Verification items for the finished model (mm, model axes). Coordinates: 2 decimals unless noted, no trailing zeros. Order: outer loops, then holes, each group sorted by start corner. A loop starts at its lowest first (then second) coordinate and runs counter-clockwise, first axis right, second up.
Q1. Thickness scan on line 1 (X direction, y = -157.5, z = 1.6); line 2 (X direction, y = -42, z = 1.55). Record the ranges inside material, lowest first.
Q2. Cross-section at A-A, the plane y = -42.5. Record the boundary of the cut face in (x, z) (3 decimals).
Q3. Cross-section at B-B, the plane x = 138. Record the boundary of the cut face in (y, z) (3 decimals), and give its area (3 significant figures).
from build123d import *

# Parameters (mm, degrees)
SKETCH1_W           = 166.124
SKETCH1_H           = 207.09
SKETCH1_R           = 3.175
BOSS_EXTRUDE1_DEPTH = 3.175


with BuildPart() as part:
    # Sketch1 → Boss-Extrude1 (new body)
    with BuildSketch(Plane.XY):
        with Locations((83.062, -103.545)):
            Rectangle(SKETCH1_W, SKETCH1_H)
        with Locations((28.287, -42.5)):
            Circle(SKETCH1_R, mode=Mode.SUBTRACT)
        with Locations(Location((137.837, -42.5, 0), (0, 0, 180))):
            Circle(SKETCH1_R, mode=Mode.SUBTRACT)
        with Locations(Location((28.287, -157.5, 0), (0, 0, 180))):
            Circle(SKETCH1_R, mode=Mode.SUBTRACT)
        with Locations((137.837, -157.5)):
            Circle(SKETCH1_R, mode=Mode.SUBTRACT)
    extrude(amount=BOSS_EXTRUDE1_DEPTH)


solid = part.part
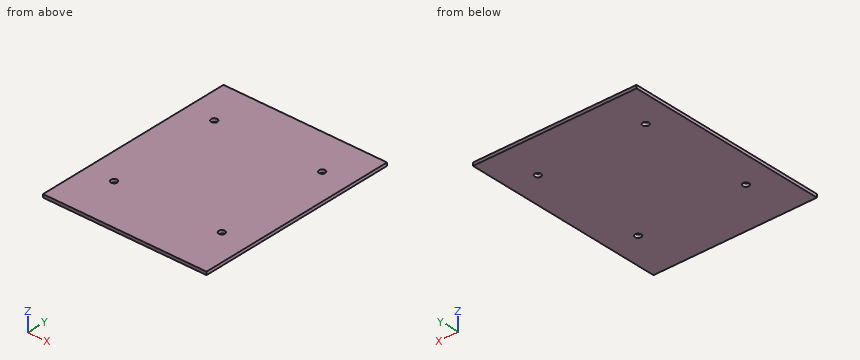
Check values:
1. line 1: x = 0 to 25.11, 31.46 to 134.66, 141.01 to 166.12
1. line 2: x = 0 to 25.15, 31.42 to 134.7, 140.97 to 166.12
2. outline: (0, 0) - (25.112, 0) - (25.112, 3.175) - (0, 3.175) - close; (31.462, 0) - (134.662, 0) - (134.662, 3.175) - (31.462, 3.175) - close; (141.012, 0) - (166.124, 0) - (166.124, 3.175) - (141.012, 3.175) - close
3. outline: (-207.09, 0) - (-160.671, 0) - (-160.671, 3.175) - (-207.09, 3.175) - close; (-154.329, 0) - (-45.671, 0) - (-45.671, 3.175) - (-154.329, 3.175) - close; (-39.329, 0) - (0, 0) - (0, 3.175) - (-39.329, 3.175) - close
3. area: 617 mm2
